Can you work these out from the model? Positions are in its coordinate system, mm. A direction names the side the tool comes from. Give positions to 0.01 mm unless a question says otherwise; leave off trailing zeros. Write each loop counter-clockwise with the first axis right and the second up, starting at its lowest first coordinate (ties: lowest second). Pieces come first, ordered by that corner, then holes.
```python
from build123d import *

# Parameters (mm, degrees)
SALIENTE_EXTRUIR1_DEPTH = 50
CROQUIS2_R              = 6
CROQUIS2_R_2            = 2.5
CORTAR_EXTRUIR1_DEPTH   = 3


with BuildPart() as part:
    # Croquis1 → Saliente-Extruir1 (new body)
    with BuildSketch(Plane.XY):
        Polygon((0, 50), (0, 0), (25, 0), (25, 3), (3, 3), (3, 50), align=None)
    extrude(amount=SALIENTE_EXTRUIR1_DEPTH)

    # Croquis2 → Cortar-Extruir1 (cut)
    with BuildSketch(Plane.ZY):
        with Locations((38, 25)):
            Circle(CROQUIS2_R)
        with Locations((38, 42.7)):
            Circle(CROQUIS2_R_2)
        with Locations((38, 7.3)):
            Circle(CROQUIS2_R_2)
    extrude(amount=-CORTAR_EXTRUIR1_DEPTH, mode=Mode.SUBTRACT)


solid = part.part
```
1) Suppose I cut it at C-C on y = 37. Write out the boundary of the cut face in (x, z).
Values follow:
outline: (0, 0) - (3, 0) - (3, 50) - (0, 50) - close
2) Suppose I cut it at B-B on z = 38. Write out the boundary of the cut face in (x, y).
Values follow:
outline: (0, 0) - (25, 0) - (25, 3) - (3, 3) - (3, 4.8) - (0, 4.8) - close; (0, 9.8) - (3, 9.8) - (3, 19) - (0, 19) - close; (0, 31) - (3, 31) - (3, 40.2) - (0, 40.2) - close; (0, 45.2) - (3, 45.2) - (3, 50) - (0, 50) - close
3) Suppose I cut it at A-A on y = 25. Write out the boundary of the cut face in (x, z).
Values follow:
outline: (0, 0) - (3, 0) - (3, 32) - (0, 32) - close; (0, 44) - (3, 44) - (3, 50) - (0, 50) - close
4) Please list where these lines run through material, in increasing order: L1, parallel to Y at x = 1.7, z = 38; L2, parallel to Y at x = 12.5, z = 17.
Values follow:
L1: y = 0 to 4.8, 9.8 to 19, 31 to 40.2, 45.2 to 50
L2: y = 0 to 3
5) Suppose I cut it at D-D on z = 12. Write out the boundary of the cut face in (x, y).
Values follow:
outline: (0, 0) - (25, 0) - (25, 3) - (3, 3) - (3, 50) - (0, 50) - close
6) If we mould it in two halves opening along Z, with no side actions, what happens to faces 1 (the face through (2, 50, 25)), 2 (the face through (1, 25, 32)), 3 (the face through (1.479, 8.051, 40.385)), 4 (the face through (2, 18, 50))? For each: +Z half, -Z half, draft (parallel to the pull), parting line (faces both ways), or undercut.
Values follow:
face 1: draft
face 2: undercut
face 3: undercut
face 4: +Z half
7) For pin 1 Ø5 at (x, y) = (11.5, 5) entering from +Z; pin 2 Ø8 at (y, z) = (23, 43) entering from +X, each with a flat end and sliding along its axis, tell me the tip position at first contact or that it passes through.
Values follow:
pin 1: stops at z = 50
pin 2: stops at x = 3
8) For faces 5 (the face through (14, 3, 25)), 6 (the face through (0, 25, 25)), which set-ups out of +Z, -Z, +X, -X, +Y, -Y let a thin tool reach every point of the face, with its end or its side?
Values follow:
face 5: +Z, -Z, +X, +Y
face 6: +Z, -Z, -X, +Y, -Y
